```python
from build123d import *

# Parameters (mm, degrees)
SKETCH1_W           = 88.4
SKETCH1_H           = 17
BOSS_EXTRUDE1_DEPTH = 1
SKETCH_1_R          = 4
CUT_EXTRUDE_1_DEPTH = 10


with BuildPart() as part:
    # Sketch1 → Boss-Extrude1 (new body)
    with BuildSketch(Plane.XY):
        with Locations((2.05547482, -11.135386556)):
            Rectangle(SKETCH1_W, SKETCH1_H)
    extrude(amount=BOSS_EXTRUDE1_DEPTH)

    # ｽｹｯﾁ1 → ｶｯﾄ - 押し出し1 (cut)
    with BuildSketch(Plane(origin=(0, 0, 0), x_dir=(-1, 0, 0), z_dir=(0, 0, -1))):
        with Locations((37.44452518, -12.985386556)):
            Circle(SKETCH_1_R)
        with BuildLine():
            Line((-12.05547482, -6.635386556), (7.94452518, -6.635386556))
            ThreePointArc((7.94452518, -6.635386556), (11.94452518, -10.635386556), (7.94452518, -14.635386556))
            Line((7.94452518, -14.635386556), (-12.05547482, -14.635386556))
            ThreePointArc((-12.05547482, -14.635386556), (-16.05547482, -10.635386556), (-12.05547482, -6.635386556))
        make_face()
    extrude(amount=-CUT_EXTRUDE_1_DEPTH, mode=Mode.SUBTRACT)


solid = part.part
```
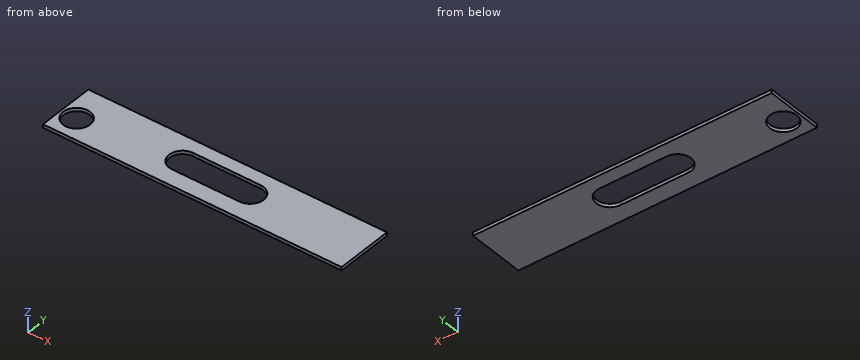
Could you check a few things on this model? Use its own coordinates, in mm. Give positions to 0.01 mm unless a question says otherwise; leave off trailing zeros. Order: outer loops, then holes, each group sorted by start corner. A loop starts at its lowest first (then second) coordinate and runs counter-clockwise, first axis right, second up.
Q1. If I drill on line 1 along Y through (x, z) = (7.5, 0.75); line 2 along X through (y, z) = (-13, 0.75); line 3 along X through (y, z) = (-9.5, 0.75), over which ranges is the centre line in solid material (lowest first)?
Q2. Suppose I cut it at B-B, the plane y = -7.75. Write out the boundary of the cut face in (x, z), and give its area (3 significant figures).
Q3. Suppose I cut it at C-C, the plane z = 0.35. Write out the boundary of the cut face in (x, y), and give its area (3 significant figures).
Q4. Suppose I cut it at A-A, the plane x = -3.5. Write out the boundary of the cut face in (y, z).
Q5. Suppose I cut it at D-D, the plane y = -11.75. Write out the boundary of the cut face in (x, z).
Solution:
1. line 1: y = -19.64 to -14.64, -6.64 to -2.64
1. line 2: x = -42.14 to -41.44, -33.44 to -11.17, 15.28 to 46.26
1. line 3: x = -42.14 to -39.41, -35.48 to -11.78, 15.89 to 46.26
2. outline: (-42.14, 0) - (-10.71, 0) - (-10.71, 1) - (-42.14, 1) - close; (14.83, 0) - (46.26, 0) - (46.26, 1) - (14.83, 1) - close
2. area: 62.9 mm2
3. outline: (-42.14, -19.64) - (46.26, -19.64) - (46.26, -2.64) - (-42.14, -2.64) - close; hole circle Ø8 at (-37.44, -12.99); hole (-7.94, -14.64) - (12.06, -14.64) arc R4 ccw to (12.06, -6.64) - (-7.94, -6.64) arc R4 ccw to start
3. area: 1,240 mm2
4. outline: (-19.64, 0) - (-14.64, 0) - (-14.64, 1) - (-19.64, 1) - close; (-6.64, 0) - (-2.64, 0) - (-2.64, 1) - (-6.64, 1) - close
5. outline: (-42.14, 0) - (-41.25, 0) - (-41.25, 1) - (-42.14, 1) - close; (-33.64, 0) - (-11.79, 0) - (-11.79, 1) - (-33.64, 1) - close; (15.9, 0) - (46.26, 0) - (46.26, 1) - (15.9, 1) - close
